```python
from build123d import *

# Parameters (mm, degrees)
SKETCH2_W           = 1000
SKETCH2_H           = 37
BOSS_EXTRUDE1_DEPTH = 35
SKETCH3_W           = 1000
SKETCH3_H           = 15
CUT_EXTRUDE1_DEPTH  = 31
SKETCH4_W           = 4
SKETCH4_H           = 35
CUT_EXTRUDE2_DEPTH  = 190


with BuildPart() as part:
    # Sketch2 → Boss-Extrude1 (new body)
    with BuildSketch(Plane(origin=(0, 0, 0), x_dir=(1, 0, 0), z_dir=(0, 1, 0))):
        with Locations((-35.123966942, 189.144628099)):
            Rectangle(SKETCH2_W, SKETCH2_H)
    extrude(amount=BOSS_EXTRUDE1_DEPTH)

    # Sketch3 → Cut-Extrude1 (cut)
    with BuildSketch(Plane(origin=(0, 35, 0), x_dir=(1, 0, 0), z_dir=(0, 1, 0))):
        with Locations((-35.123966942, 198.144628099)):
            Rectangle(SKETCH3_W, SKETCH3_H)
        with Locations((-35.123966942, 180.144628099)):
            Rectangle(SKETCH3_W, SKETCH3_H)
    extrude(amount=-CUT_EXTRUDE1_DEPTH, mode=Mode.SUBTRACT)

    # Sketch4 → Cut-Extrude2 (cut)
    with BuildSketch(Plane(origin=(0, 0, -207.644628099), x_dir=(-1, 0, 0), z_dir=(0, 0, -1))):
        with Locations((533.123966942, 17.5)):
            Rectangle(SKETCH4_W, SKETCH4_H)
    extrude(amount=-CUT_EXTRUDE2_DEPTH, mode=Mode.SUBTRACT)


solid = part.part
```
Geometry check sheet. Reference: the model listing, model coordinates, mm. A direction names the side the tool comes from. Give positions to 0.01 mm unless a question says otherwise; leave off trailing zeros. Write each loop counter-clockwise with the first axis right and the second up, starting at its lowest first coordinate (ties: lowest second). Pieces come first, ordered by that corner, then holes.
1) Section check B-B, the plane x = -343. Record the boundary of the cut face in (y, z), and give its area (3 significant figures).
2) Section check C-C, the plane z = -182. Record the boundary of the cut face in (x, y), and give its area (3 significant figures).
3) Section check A-A, the plane y = 9.5. Record the boundary of the cut face in (x, z), and give its area (3 significant figures).
4) Gauge pin test, flat end, axial feed: pin 1 (12 mm diameter, centred on x = 144, z = -198, fed in from +Y). Record the tip position at first contact, or that the pin passes through.
5) Material ranges on L1, parallel to Z at x = -385, y = 23.5; L2, parallel to Y at x = 226, z = -193, recorded low to high.
6) Access from +Z, -Z, +X, -X, +Y, -Y to the whole of each face (thin tool, end or side, straight path). Record for faces 1 (the flat face through (-40, 17, -170.645)), 2 (the flat face through (-40, 20, -190.645)).
Computed:
1. outline: (0, -207.64) - (35, -207.64) - (35, -205.64) - (4, -205.64) - (4, -190.64) - (35, -190.64) - (35, -187.64) - (4, -187.64) - (4, -172.64) - (35, -172.64) - (35, -170.64) - (0, -170.64) - close
1. area: 365 mm2
2. outline: (-531.12, 0) - (464.88, 0) - (464.88, 4) - (-531.12, 4) - close
2. area: 3,980 mm2
3. outline: (-531.12, -207.64) - (464.88, -207.64) - (464.88, -205.64) - (-531.12, -205.64) - close; (-531.12, -190.64) - (464.88, -190.64) - (464.88, -187.64) - (-531.12, -187.64) - close; (-531.12, -172.64) - (464.88, -172.64) - (464.88, -170.64) - (-531.12, -170.64) - close
3. area: 6,970 mm2
4. pin 1: stops at y = 4
5. L1: z = -207.64 to -205.64, -190.64 to -187.64, -172.64 to -170.64
5. L2: y = 0 to 4
6. face 1: +Z, +X, -X, +Y, -Y
6. face 2: +X, -X, +Y
